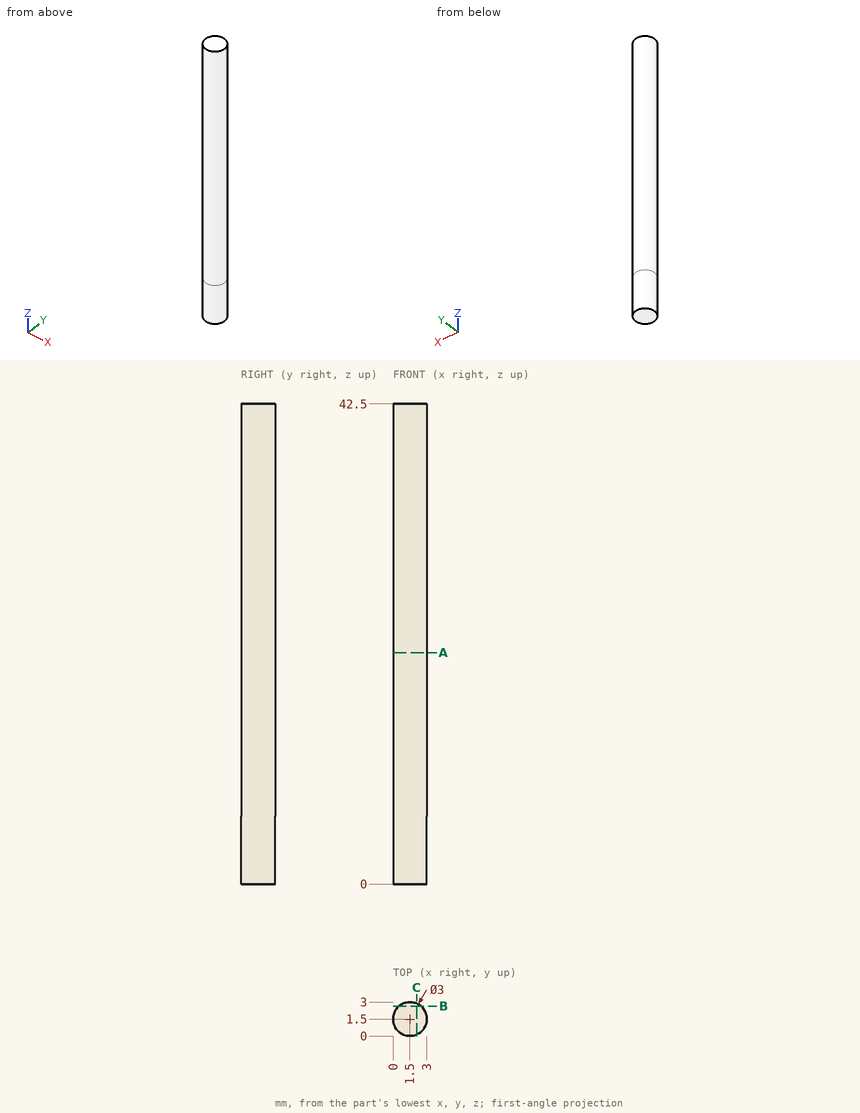
Source: three-view drawing plus pictorial views. Frame: mm from the lowest corner of the part. Round coordinates to 2 decimals unless told otherwise and drop trailing zeros. Order: outer loops, then holes, each group sorted by start corner. A loop starts at its lowest first (then second) coordinate and runs counter-clockwise, first axis right, second up. Notation, with made-up numbers: (2.5, -8.75) -> (19.5, -8.75) arc R18 ccw to (19.5, 19.25) -> close; hole circle Ø2 at (-2, 73.5). An arc over 180 degrees is marked (long way). Use one line per item in the form item = value.
(1) Section B-B on y = 2.65. Return loops of the section in (x, z).
Results list:
outline = (0.54, 0) -> (2.46, 0) -> (2.46, 42.5) -> (0.54, 42.5) -> close
(2) Section C-C on x = 2.1. Return loops of the section in (y, z).
Results list:
outline = (0.13, 0) -> (2.87, 0) -> (2.87, 42.5) -> (0.13, 42.5) -> close
(3) Section A-A on z = 20.5. Return loops of the section in (x, y).
Results list:
outline = circle Ø3 at (1.5, 1.5)
(4) Ray query, probe 1 along X at (y, z) = (1.6, 22); probe 2 along X at (y, z) = (2.25, 29.5). Return the intervals inside material, ascending. Write a range as [from, to].
Results list:
probe_1 = [0, 3]
probe_2 = [0.2, 2.8]
